Check sheet for the modelled part. Datum: model origin and axes. Units: mm. A direction names the side the tool comes from. Round coordinates to 2 decimals unless told otherwise and drop trailing zeros. Write each loop counter-clockwise with the first axis right and the second up, starting at its lowest first coordinate (ties: lowest second). Pieces come first, ordered by that corner, then holes.
Item 1: Section check D-D, the plane y = -9.25. Record the cut outline in (x, z), plus the area to 3 significant figures.
Item 2: Depth check by flat-ended pin: pin 1 (12 mm diameter, centred on x = -6.5, y = 3.5, fed in from -Z); pin 2 (1.5 mm diameter, centred on x = -7, z = -19, fed in from -Y); pin 3 (12 mm diameter, centred on y = 7, z = -10, fed in from +X); pin 4 (4 mm diameter, centred on y = -6, z = -40, fed in from -X). Enter the tip coordinate at first touch or a pass-through.
Item 3: Material ranges on line 1 along Y through (x, z) = (0, -29); line 2 along X through (y, z) = (-0.5, 16); line 3 along Z through (x, y) = (7, 3.75), recorded low to high.
Item 4: Section check C-C, the plane z = 38. Record the cut outline in (x, y).
Item 5: Set-up check for faces 4 (the cylindrical face through (-7.89, 0.35, 0.89)), 5 (the flat face through (6.454, 6.655, -39.665)): record each of +Z, -Z, +X, -X, +Y, -Y from which the full face is reachable in a straight line by a thin tool's end or side.
Item 6: Section check B-B, the plane y = -2.75. Record the cut outline in (x, z), plus the area to 3 significant figures.
Item 7: Release check for a two-part mould opening along X. For faces 1 (the flat face through (9.256, 0.522, 10.1)), 2 (the flat face through (-7, -4, 63.5)), 3 (the flat face through (7.89, 4.92, 10.16)) record: pulls with the +X half, pulls with the -X half, needs draft (parallel to the pull), parting line crosses it, or undercut.
Item 8: Section check A-A, the plane x = 0. Record the cut outline in (y, z).
Autodesk Inventor part; units mm, degrees
ref_plane "YZ Plane" through (0, 0, 0) normal (1, 0, 0) x (0, 1, 0)
ref_plane "XZ Plane" through (0, 0, 0) normal (0, 1, 0) x (-1, 0, 0)
ref_plane "XY Plane" through (0, 0, 0) normal (0, 0, 1) x (1, 0, 0)
sketch "Sketch1" plane through (0, 0, 0) normal (0, 0, 1) x (1, 0, 0)
  circle A0 centre (0, 0) radius 7.8994
  circle A1 centre (0, 0) radius 10.668
  dimension "d0" = 15.7988
  dimension "d2" = 21.336
extrude "Extrusion1" add sketch "Sketch1" along normal mid plane 127
ref_plane "Work Plane1" through (0, 0, -38.1) normal (0, 0, -1) x (-1, 0, 0)
sketch "Sketch3" plane through (0, 0, -38.1) normal (0, 0, -1) x (-1, 0, 0)
  line L0 (-7.3505, 7.6359) -> (-5.5315, 5.6464)
  line L1 (-5.5315, 5.6464) -> (-7.3505, 7.6359)
  line L2 (-6.8389, 3.8843) -> (-9.0558, 5.6464)
  arc A0 (-7.3505, 7.6359) -> (-9.0558, 5.6464) centre (5.6213, -5.2084) ccw
  arc A1 (-5.5315, 5.6464) -> (-6.8389, 3.8843) centre (-5.2401, 4.0642) ccw
  point P0 (0, 0)
extrude "Extrusion3" cut sketch "Sketch3" along normal blind 3.175
ref_plane "Work Plane3" through (9.0527, 5.644, 0) normal (0.8486, 0.5291, 0) x (-0.5291, 0.8486, 0)
sketch "Sketch4" plane through (9.0527, 5.644, 0) normal (0.8486, 0.5291, 0) x (-0.5291, 0.8486, 0)
  line L0 (0, 12.2855) -> (0, 7.9748)
  line L1 (0, 7.9748) -> (-4.4544, 7.9748)
  line L2 (-4.4544, 7.9748) -> (-4.4544, 12.2855)
  line L3 (-4.4544, 12.2855) -> (0, 12.2855)
  point P0 (0, 0)
extrude "Extrusion4" cut sketch "Sketch4" against normal blind 6.35
properties part number "PVC Spacer 500 Sched 40" material "PVC-Piping"
Values found:
1. outline: (-5.31, -63.5) - (5.31, -63.5) - (5.31, 63.5) - (-5.31, 63.5) - close
1. area: 1,350 mm2
2. pin 1: stops at z = -63.5
2. pin 2: stops at y = -8.65
2. pin 3: stops at x = 10.62
2. pin 4: stops at x = -9.89
3. line 1: y = -10.67 to -7.9, 7.9 to 10.67
3. line 2: x = -10.66 to -7.88, 7.88 to 10.66
3. line 3: z = -63.5 to 7.97, 12.29 to 63.5
4. outline: circle Ø21.34 at (0, 0); hole circle Ø15.8 at (0, 0)
5. face 4: +Z, -Z
5. face 5: none
6. outline: (-10.31, -63.5) - (-7.41, -63.5) - (-7.41, 63.5) - (-10.31, 63.5) - close; (7.41, -63.5) - (10.31, -63.5) - (10.31, 63.5) - (7.41, 63.5) - close
6. area: 737 mm2
7. face 1: undercut
7. face 2: needs draft
7. face 3: pulls with the +X half
8. outline: (-10.67, -63.5) - (-7.9, -63.5) - (-7.9, 63.5) - (-10.67, 63.5) - close; (7.9, -63.5) - (10.67, -63.5) - (10.67, 63.5) - (7.9, 63.5) - close
